Source: CAD feature listing. Evaluate the final solid. Frame: model axes, mm. Face numbers are marked on the shaded views. A direction names the side the tool comes from. Round coordinates to 2 decimals unless told otherwise and drop trailing zeros. Order: outer loops, then holes, each group sorted by start corner. A loop starts at its lowest first (then second) coordinate and runs counter-clockwise, first axis right, second up. Notation, with made-up numbers: (47.5, -33) -> (59.5, -33) arc R28 ccw to (59.5, -9) -> close; hole circle Ø10 at (48, 39). An arc over 180 degrees is marked (long way). Answer as CSV lines item,"result". Start each with the question number.
(1) Set-up query: the marked faces 1 and 2. Return all of +Z, -Z, +X, -X, +Y, -Y with unobstructed straight access to the full face (end or side cutting, diameter ignored); none if empty.
(2) Pull-direction query (X, two-part tool) for the marked faces 3, 4 and 5; classes: +X half, -X half, draft (parallel to the pull), parting line (faces both ways), or undercut.
(3) Line query: line 1 along X through (y, z) = (0.25, 3); line 2 along Y through (x, z) = (-4.75, 12.75); line 3 along Z through (x, y) = (-4.75, 3.75). Output: solid intervals per line, ascending. Write a range as from..to.
(4) Section query D-D (z = 5). Output: boundary loops of the cut face in (x, y), plus the area to 3 significant figures.
(5) Section query A-A (z = 3). Output: boundary loops of the cut face in (x, y).
(6) Section query B-B (y = 2). Output: boundary loops of the cut face in (x, z).
(7) Section query C-C (y = 3.5). Output: boundary loops of the cut face in (x, z), plus the area to 3 significant figures.
```python
from build123d import *

# Parameters (mm, degrees)
SKETCH1_W                     = 7.5
SKETCH1_H                     = 10
BOSS_EXTRUDE1_DEPTH           = 15
HOLE_FOR_TUBING_R             = 1.1
CUT_EXTRUDE1_DEPTH            = 16
F_10_32_HOLE_FOR_LUER_SCREW_R = 2.0193
CUT_EXTRUDE2_DEPTH            = 7.5
F_4_40_SET_SCREW_HOLE_R       = 1.1303
CUT_EXTRUDE3_DEPTH            = 11


with BuildPart() as part:
    # Sketch1 → Boss-Extrude1 (new body)
    with BuildSketch(Plane.XY):
        with Locations((-4.663043478, 2.239130435)):
            Rectangle(SKETCH1_W, SKETCH1_H)
    extrude(amount=BOSS_EXTRUDE1_DEPTH)

    # hole for tubing → Cut-Extrude1 (cut, through all)
    with BuildSketch(Plane(origin=(0, 0, 0), x_dir=(-1, 0, 0), z_dir=(0, 0, -1))):
        with Locations((4.663043478, 2.239130435)):
            Circle(HOLE_FOR_TUBING_R)
    extrude(amount=-CUT_EXTRUDE1_DEPTH, mode=Mode.SUBTRACT)

    # 10-32 hole for luer screw → Cut-Extrude2 (cut)
    with BuildSketch(Plane.XY.offset(15)):
        with Locations((-4.663043478, 2.239130435)):
            Circle(F_10_32_HOLE_FOR_LUER_SCREW_R)
    extrude(amount=-CUT_EXTRUDE2_DEPTH, mode=Mode.SUBTRACT)

    # 4-40 set screw hole → Cut-Extrude3 (cut, through all)
    with BuildSketch(Plane(origin=(0, 7.239130435, 0), x_dir=(1, 0, 0), z_dir=(0, 1, 0))):
        with Locations((-4.663043478, -3)):
            Circle(F_4_40_SET_SCREW_HOLE_R)
    extrude(amount=-CUT_EXTRUDE3_DEPTH, mode=Mode.SUBTRACT)


solid = part.part
```
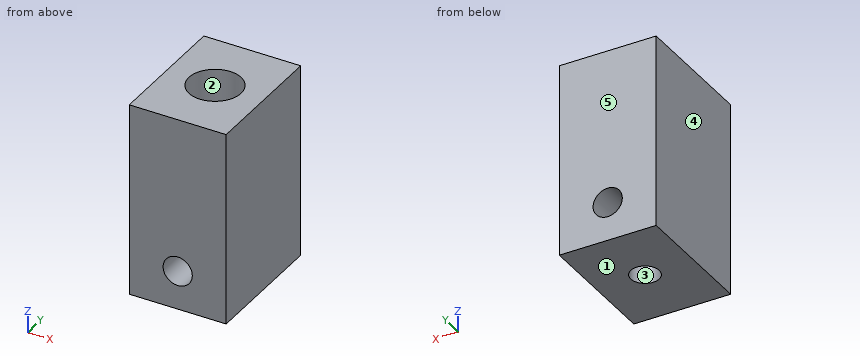
Answer block:
1,face 1,"-Z, +X, -X, +Y, -Y"
1,face 2,"+Z"
2,face 3,"undercut"
2,face 4,"-X half"
2,face 5,"draft"
3,line 1,"-8.41..-5.79, -3.53..-0.91"
3,line 2,"-2.76..0.22, 4.26..7.24"
3,line 3,"0..1.87, 4.13..7.5"
4,outline,"(-8.41, -2.76) -> (-0.91, -2.76) -> (-0.91, 7.24) -> (-8.41, 7.24) -> close; hole circle Ø2.2 at (-4.66, 2.24)"
4,area,"71.2 mm2"
5,outline,"(-8.41, -2.76) -> (-5.79, -2.76) -> (-5.79, 7.24) -> (-8.41, 7.24) -> close; (-3.53, -2.76) -> (-0.91, -2.76) -> (-0.91, 7.24) -> (-3.53, 7.24) -> close"
6,outline,"(-8.41, 0) -> (-5.74, 0) -> (-5.74, 2.65) arc R1.13 cw to (-5.74, 3.35) -> (-5.74, 7.5) -> (-6.67, 7.5) -> (-6.67, 15) -> (-8.41, 15) -> close; (-3.59, 0) -> (-0.91, 0) -> (-0.91, 15) -> (-2.66, 15) -> (-2.66, 7.5) -> (-3.59, 7.5) -> (-3.59, 3.35) arc R1.13 cw to (-3.59, 2.65) -> close"
7,outline,"(-8.41, 0) -> (-0.91, 0) -> (-0.91, 15) -> (-3.09, 15) -> (-3.09, 7.5) -> (-6.24, 7.5) -> (-6.24, 15) -> (-8.41, 15) -> close; hole circle Ø2.26 at (-4.66, 3)"
7,area,"84.8 mm2"
